Design review of the part shown in the three views and the two pictorial views. Dimensions are in mm from the part's minimum x, y and z. A direction names the side the tool comes from. Round coordinates to 2 decimals unless told otherwise and drop trailing zeros. Loops run counter-clockwise (first coordinate to the right, second up) from the corner with the lowest first, then second, coordinate; pieces in that order, holes last. Notation, with made-up numbers: M 16,-14.5 L 28,-14.5 A24 cw 28,23.5 Z; hole C -39.5,18 d3. An arc over 180 degrees is marked long. Return JSON: item names as keys, results as strings. Group by question number.
Q1. Draft analysis for pull direction Z (two halves, no side actions). For the marked faces 4, 5 and 6, state which applies: pulls with the +Z half, pulls with the -Z half, needs draft (parallel to the pull), parting line crosses it, or undercut.
Q2. Consider section B-B (x = 139.7). State the section outline as (y, z) points.
Q3. Consider section A-A (z = 195.5). State the section outline as (x, y) points.
Q4. For the marked faces 1, 2 and 3, list the 3-axis set-ups (+Z, -Z, +X, -X, +Y, -Y) from which the entire face can be reached by the end or side of a thin tool; tool diameter is ignored.
Q5. Consider section D-D (x = 178). State the section outline as (y, z) points, and give its area (3 significant figures).
Q6. To check wall thickness, follow line 1 along Z through (x, y) = (158, 12.25); line 2 along Z through (x, y) = (175.5, 4.5) (3 decimals); line 3 along Z through (x, y) = (246.5, 1.75). State the ranges of each line that lie inside material, in increasing order.
Q7. Clearance check with flat-ended pins moving along their axes: pin 1 Ø7.5 at (x, y) = (179, 16.5) entering from -Z; pin 2 Ø8 at (x, y) = (238, 16) entering from -Z; pin 3 Ø3 at (y, z) = (22, 216.5) entering from +X. State where each tip first meets the part, or that it passes through.
Q8. Consider section C-C (y = 18.5). State the section outline as (x, z) points.
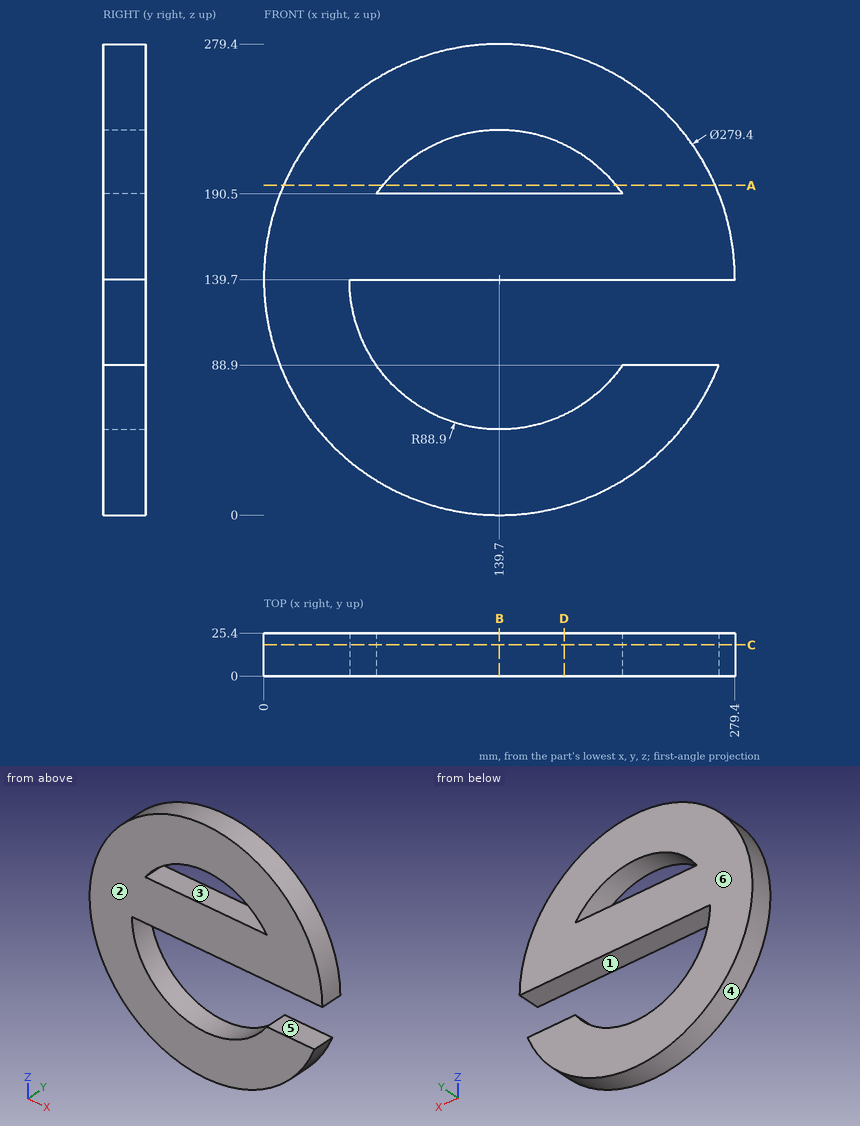
Values:
{
 "1": {"face 4": "parting line crosses it", "face 5": "undercut", "face 6": "needs draft"},
 "2": {"outline": "M 0,0 L 25.4,0 L 25.4,50.8 L 0,50.8 Z; M 0,139.7 L 25.4,139.7 L 25.4,190.5 L 0,190.5 Z; M 0,228.6 L 25.4,228.6 L 25.4,279.4 L 0,279.4 Z"},
 "3": {"outline": "M 11.63,0 L 70.49,0 L 70.49,25.4 L 11.63,25.4 Z; M 208.91,0 L 267.77,0 L 267.77,25.4 L 208.91,25.4 Z"},
 "4": {"face 1": "+X, +Y, -Y", "face 2": "+Z, -Z, +X, -X, -Y", "face 3": "+Y, -Y"},
 "5": {"outline": "M 0,5.35 L 25.4,5.35 L 25.4,59.47 L 0,59.47 Z; M 0,139.7 L 25.4,139.7 L 25.4,190.5 L 0,190.5 Z; M 0,219.93 L 25.4,219.93 L 25.4,274.05 L 0,274.05 Z", "area": "4,040 mm2"},
 "6": {"line 1": "z = 1.2 to 52.7, 139.7 to 190.5, 226.7 to 278.2", "line 2": "z = 4.665 to 58.327, 139.7 to 190.5, 221.073 to 274.735", "line 3": "z = 49.65 to 88.9, 139.7 to 229.75"},
 "7": {"pin 1": "stops at z = 4.6", "pin 2": "stops at z = 36.63", "pin 3": "stops at x = 257.37"},
 "8": {"outline": "M 50.8,139.7 L 279.4,139.7 A139.7 ccw long 269.84,88.9 L 212.66,88.9 A88.9 cw Z; hole M 66.74,190.5 L 212.66,190.5 A88.9 ccw Z"}
}
